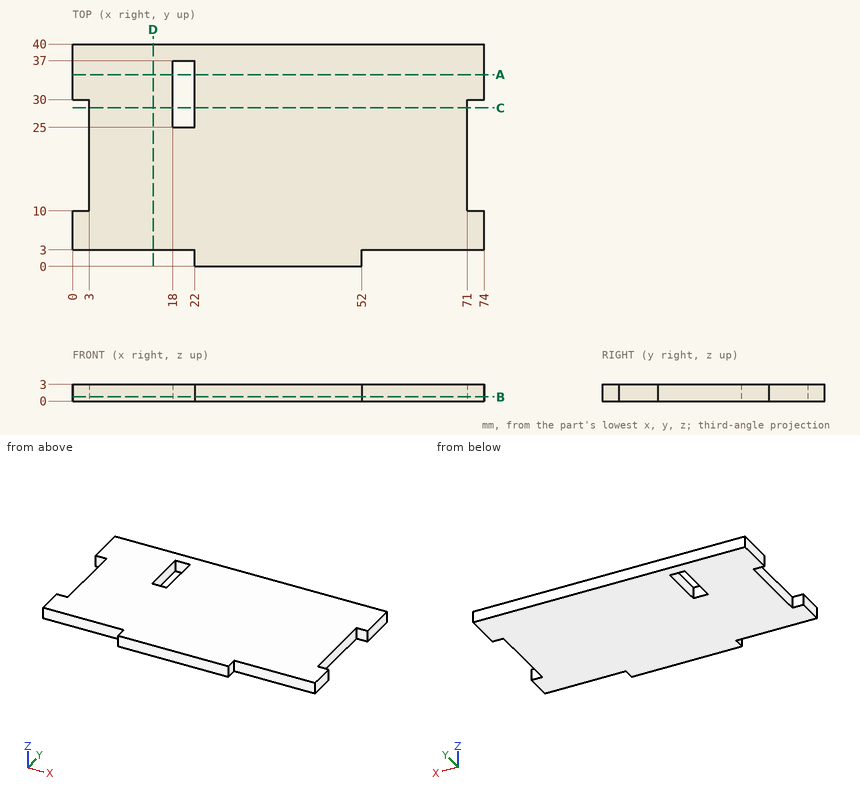
Design review of the part shown in the three views and the two pictorial views. Dimensions are in mm from the part's minimum x, y and z. Give positions to 0.01 mm unless a question says otherwise; leave off trailing zeros. Write each loop counter-clockwise with the first axis right and the second up, starting at its lowest first coordinate (ties: lowest second). Pieces come first, ordered by that corner, then holes. Notation, with made-up numbers: M 86,71 L 98,71 A22 cw 98,93 Z; hole C -25,70.25 d6. An arc over 180 degrees is marked long. Answer in a Markdown table with one row per item.
Item 1: Add section C-C on y = 28.5. Give the boundary of the cut face in (x, z), plus the area to 3 significant figures.
Check sheet entries:
| item | result |
|---|---|
| outline | M 3,0 L 18,0 L 18,3 L 3,3 Z; M 22,0 L 71,0 L 71,3 L 22,3 Z |
| area | 192 mm2 |
Item 2: Add section B-B on z = 0.75. Give the boundary of the cut face in (x, y).
Check sheet entries:
| item | result |
|---|---|
| outline | M 0,3 L 22,3 L 22,0 L 52,0 L 52,3 L 74,3 L 74,10 L 71,10 L 71,30 L 74,30 L 74,40 L 0,40 L 0,30 L 3,30 L 3,10 L 0,10 Z; hole M 18,25 L 22,25 L 22,37 L 18,37 Z |
Item 3: For line 1 along X through (y, z) = (33.5, 0.3); line 2 along X through (y, z) = (29, 1.45); line 3 along Y through (x, z) = (5, 1.1), list the stretches that pass through material, from the lowest coordinate up.
Check sheet entries:
| item | result |
|---|---|
| line 1 | 0 to 18, 22 to 74 |
| line 2 | 3 to 18, 22 to 71 |
| line 3 | 3 to 40 |
Item 4: Add section A-A on y = 34.5. Give the boundary of the cut face in (x, z), plus the area to 3 significant figures.
Check sheet entries:
| item | result |
|---|---|
| outline | M 0,0 L 18,0 L 18,3 L 0,3 Z; M 22,0 L 74,0 L 74,3 L 22,3 Z |
| area | 210 mm2 |
Item 5: Add section D-D on x = 14.5. Give the boundary of the cut face in (y, z).
Check sheet entries:
| item | result |
|---|---|
| outline | M 3,0 L 40,0 L 40,3 L 3,3 Z |
Item 6: For P1, Ø0.9, axis at x = 66, z = 2, coming from the -Y side; P2, Ø1.5, axis at y = 18.5, z = 2, coming from the -X side, all flat-tipped, find the tip position at first contact; note any pin that passes through.
Check sheet entries:
| item | result |
|---|---|
| P1 | y = 3 |
| P2 | x = 3 |
